from build123d import *

# Parameters (mm, degrees)
ESBO_O1_W                        = 48
ESBO_O1_H                        = 124
FLANGE_BASE1_DEPTH               = 2
ARESTA_FLANGE1_STRIP_W           = 10
ARESTA_FLANGE1_STRIP_H           = 2
ARESTA_FLANGE1_STRIP_CUT_DEPTH   = 48
ARESTA_FLANGE1_STRIP_2_W         = 10
ARESTA_FLANGE1_STRIP_2_H         = 2
ARESTA_FLANGE1_STRIP_CUT_2_DEPTH = 48
ARESTA_FLANGE1_DEPTH             = 48
ARESTA_FLANGE1_BEND_DEPTH        = 48
CORTE_EXTRUS_O1_REACH            = 151.295
ESBO_O14_R                       = 1.25
ESBO_O15_R                       = 6.5
CORTE_EXTRUS_O2_DEPTH            = 2
FILETE1_R                        = 4
ESBO_O16_R                       = 3
ESBO_O16_R_2                     = 1.25
CORTE_EXTRUS_O3_DEPTH            = 2


# Sheet-metal steps are written as plain solids
with BuildPart() as part:
    # Esboço1 → Flange-base1 (new body)
    with BuildSketch(Plane(origin=(0, 0, 0), x_dir=(1, 0, 0), z_dir=(0, 1, 0))):
        Rectangle(ESBO_O1_W, ESBO_O1_H)
    extrude(amount=-FLANGE_BASE1_DEPTH)

    # Aresta-Flange1 strip (across the edge) → Aresta-Flange1 strip cut (cut)
    with BuildSketch(Plane(origin=(-24, 0, 62), x_dir=(0, 0, -1), z_dir=(1, 0, 0))):
        with Locations((-4, -1)):
            Rectangle(ARESTA_FLANGE1_STRIP_W, ARESTA_FLANGE1_STRIP_H)
    extrude(amount=ARESTA_FLANGE1_STRIP_CUT_DEPTH, mode=Mode.SUBTRACT)

    # Aresta-Flange1 strip 2 (across the edge) → Aresta-Flange1 strip cut 2 (cut)
    with BuildSketch(Plane(origin=(24, 0, -62), x_dir=(0, 0, 1), z_dir=(-1, 0, 0))):
        with Locations((-4, -1)):
            Rectangle(ARESTA_FLANGE1_STRIP_2_W, ARESTA_FLANGE1_STRIP_2_H)
    extrude(amount=ARESTA_FLANGE1_STRIP_CUT_2_DEPTH, mode=Mode.SUBTRACT)

    # Aresta-Flange1 section (across the edge) → Aresta-Flange1 (add)
    with BuildSketch(Plane(origin=(-24, 0, 62), x_dir=(0, 0, -1), z_dir=(1, 0, 0))):
        with BuildLine():
            Line((-2, 1), (-2, 73))
            Line((-2, 73), (0, 73))
            Line((0, 73), (0, 1))
            ThreePointArc((0, 1), (0.292893219, 0.292893219), (1, 0))
            Line((1, 0), (1, -2))
            ThreePointArc((1, -2), (-1.121320344, -1.121320344), (-2, 1))
        make_face()
    extrude(amount=ARESTA_FLANGE1_DEPTH)

    # Aresta-Flange1 section 2 (across the edge) → Aresta-Flange1 bend (add)
    with BuildSketch(Plane(origin=(24, 0, -62), x_dir=(0, 0, 1), z_dir=(-1, 0, 0))):
        with BuildLine():
            Line((-2, 1), (-2, 73))
            Line((-2, 73), (0, 73))
            Line((0, 73), (0, 1))
            ThreePointArc((0, 1), (0.292893219, 0.292893219), (1, 0))
            Line((1, 0), (1, -2))
            ThreePointArc((1, -2), (-1.121320344, -1.121320344), (-2, 1))
        make_face()
    extrude(amount=ARESTA_FLANGE1_BEND_DEPTH)

    # Corte-extrusão1: up to this face of the body (flat: up to its plane)
    corte_extrus_o1_end = Plane(part.part.faces().sort_by_distance((0, 37, -64))[0])
    # Esboço14 → Corte-extrusão1 (cut, up to the picked face)
    with BuildSketch(Plane.XY.offset(64), mode=Mode.PRIVATE) as corte_extrus_o1_sk1:
        with Locations(Location((-11, 62, 0), (0, 0, 180))):
            Circle(ESBO_O14_R)
    corte_extrus_o1_tool1 = split(extrude(corte_extrus_o1_sk1.sketch, amount=-CORTE_EXTRUS_O1_REACH, mode=Mode.PRIVATE), bisect_by=corte_extrus_o1_end, keep=Keep.BOTH, mode=Mode.PRIVATE)
    # Esboço14 → Corte-extrusão1 (cut, up to the picked face)
    with BuildSketch(Plane.XY.offset(64), mode=Mode.PRIVATE) as corte_extrus_o1_sk2:
        with Locations(Location((-7.778174593, 69.778174593, 0), (0, 0, 270))):
            Circle(ESBO_O14_R)
    corte_extrus_o1_tool2 = split(extrude(corte_extrus_o1_sk2.sketch, amount=-CORTE_EXTRUS_O1_REACH, mode=Mode.PRIVATE), bisect_by=corte_extrus_o1_end, keep=Keep.BOTH, mode=Mode.PRIVATE)
    # Esboço14 → Corte-extrusão1 (cut, up to the picked face)
    with BuildSketch(Plane.XY.offset(64), mode=Mode.PRIVATE) as corte_extrus_o1_sk3:
        with Locations(Location((7.778174593, 69.778174593, 0), (0, 0, 270))):
            Circle(ESBO_O14_R)
    corte_extrus_o1_tool3 = split(extrude(corte_extrus_o1_sk3.sketch, amount=-CORTE_EXTRUS_O1_REACH, mode=Mode.PRIVATE), bisect_by=corte_extrus_o1_end, keep=Keep.BOTH, mode=Mode.PRIVATE)
    # Esboço14 → Corte-extrusão1 (cut, up to the picked face)
    with BuildSketch(Plane.XY.offset(64), mode=Mode.PRIVATE) as corte_extrus_o1_sk4:
        with Locations(Location((11, 62, 0), (0, 0, 270))):
            Circle(ESBO_O14_R)
    corte_extrus_o1_tool4 = split(extrude(corte_extrus_o1_sk4.sketch, amount=-CORTE_EXTRUS_O1_REACH, mode=Mode.PRIVATE), bisect_by=corte_extrus_o1_end, keep=Keep.BOTH, mode=Mode.PRIVATE)
    # Esboço14 → Corte-extrusão1 (cut, up to the picked face)
    with BuildSketch(Plane.XY.offset(64), mode=Mode.PRIVATE) as corte_extrus_o1_sk5:
        with Locations(Location((7.778174593, 54.221825407, 0), (0, 0, 270))):
            Circle(ESBO_O14_R)
    corte_extrus_o1_tool5 = split(extrude(corte_extrus_o1_sk5.sketch, amount=-CORTE_EXTRUS_O1_REACH, mode=Mode.PRIVATE), bisect_by=corte_extrus_o1_end, keep=Keep.BOTH, mode=Mode.PRIVATE)
    # Esboço14 → Corte-extrusão1 (cut, up to the picked face)
    with BuildSketch(Plane.XY.offset(64), mode=Mode.PRIVATE) as corte_extrus_o1_sk6:
        with Locations(Location((0, 51, 0), (0, 0, 270))):
            Circle(ESBO_O14_R)
    corte_extrus_o1_tool6 = split(extrude(corte_extrus_o1_sk6.sketch, amount=-CORTE_EXTRUS_O1_REACH, mode=Mode.PRIVATE), bisect_by=corte_extrus_o1_end, keep=Keep.BOTH, mode=Mode.PRIVATE)
    # Esboço14 → Corte-extrusão1 (cut, up to the picked face)
    with BuildSketch(Plane.XY.offset(64), mode=Mode.PRIVATE) as corte_extrus_o1_sk7:
        with Locations(Location((-7.778174593, 54.221825407, 0), (0, 0, 270))):
            Circle(ESBO_O14_R)
    corte_extrus_o1_tool7 = split(extrude(corte_extrus_o1_sk7.sketch, amount=-CORTE_EXTRUS_O1_REACH, mode=Mode.PRIVATE), bisect_by=corte_extrus_o1_end, keep=Keep.BOTH, mode=Mode.PRIVATE)
    # Esboço14 → Corte-extrusão1 (cut, up to the picked face)
    with BuildSketch(Plane.XY.offset(64), mode=Mode.PRIVATE) as corte_extrus_o1_sk8:
        with BuildLine():
            Line((-5, 62), (-5, 73))
            Line((-5, 73), (5, 73))
            Line((5, 73), (5, 62))
            ThreePointArc((5, 62), (0, 57), (-5, 62))
        make_face()
    corte_extrus_o1_tool8 = split(extrude(corte_extrus_o1_sk8.sketch, amount=-CORTE_EXTRUS_O1_REACH, mode=Mode.PRIVATE), bisect_by=corte_extrus_o1_end, keep=Keep.BOTH, mode=Mode.PRIVATE)
    # Esboço14 → Corte-extrusão1 (cut, up to the picked face)
    with BuildSketch(Plane.XY.offset(64), mode=Mode.PRIVATE) as corte_extrus_o1_sk9:
        Polygon((-24, 1), (-12, 68.528174593), (-9, 73), (-24, 73), align=None)
    corte_extrus_o1_tool9 = split(extrude(corte_extrus_o1_sk9.sketch, amount=-CORTE_EXTRUS_O1_REACH, mode=Mode.PRIVATE), bisect_by=corte_extrus_o1_end, keep=Keep.BOTH, mode=Mode.PRIVATE)
    # Esboço14 → Corte-extrusão1 (cut, up to the picked face)
    with BuildSketch(Plane.XY.offset(64), mode=Mode.PRIVATE) as corte_extrus_o1_sk10:
        Polygon((24, 73), (9, 73), (12, 68.528174593), (24, 1), align=None)
    corte_extrus_o1_tool10 = split(extrude(corte_extrus_o1_sk10.sketch, amount=-CORTE_EXTRUS_O1_REACH, mode=Mode.PRIVATE), bisect_by=corte_extrus_o1_end, keep=Keep.BOTH, mode=Mode.PRIVATE)
    add(corte_extrus_o1_tool1.solids().sort_by(Axis((-11, 62, 64), (0, 0, -1)))[0], mode=Mode.SUBTRACT)
    add(corte_extrus_o1_tool2.solids().sort_by(Axis((-7.778175, 69.778175, 64), (0, 0, -1)))[0], mode=Mode.SUBTRACT)
    add(corte_extrus_o1_tool3.solids().sort_by(Axis((7.778175, 69.778175, 64), (0, 0, -1)))[0], mode=Mode.SUBTRACT)
    add(corte_extrus_o1_tool4.solids().sort_by(Axis((11, 62, 64), (0, 0, -1)))[0], mode=Mode.SUBTRACT)
    add(corte_extrus_o1_tool5.solids().sort_by(Axis((7.778175, 54.221825, 64), (0, 0, -1)))[0], mode=Mode.SUBTRACT)
    add(corte_extrus_o1_tool6.solids().sort_by(Axis((0, 51, 64), (0, 0, -1)))[0], mode=Mode.SUBTRACT)
    add(corte_extrus_o1_tool7.solids().sort_by(Axis((-7.778175, 54.221825, 64), (0, 0, -1)))[0], mode=Mode.SUBTRACT)
    add(corte_extrus_o1_tool8.solids().sort_by(Axis((0, 65.494788, 64), (0, 0, -1)))[0], mode=Mode.SUBTRACT)
    add(corte_extrus_o1_tool9.solids().sort_by(Axis((-19.639786, 49.238418, 64), (0, 0, -1)))[0], mode=Mode.SUBTRACT)
    add(corte_extrus_o1_tool10.solids().sort_by(Axis((19.639786, 49.238418, 64), (0, 0, -1)))[0], mode=Mode.SUBTRACT)

    # Esboço15 → Corte-extrusão2 (cut)
    with BuildSketch(Plane(origin=(0, 0, 0), x_dir=(1, 0, 0), z_dir=(0, 1, 0))):
        with Locations(Location((0, -30, 0), (0, 0, 270))):
            Circle(ESBO_O15_R)
        with Locations(Location((0, 30, 0), (0, 0, 270))):
            Circle(ESBO_O15_R)
    extrude(amount=-CORTE_EXTRUS_O2_DEPTH, mode=Mode.SUBTRACT)

    # Filete1
    # the kernel refuses this fillet: 4 mm, written as the material it takes off along each edge
    with BuildSketch(Plane(origin=(-12, 68.528174593, -59.894503429), x_dir=(-0.17496254204261552, -0.9845750905248344, 0), z_dir=(0, 0, -1)), Plane(origin=(-12, 68.528174593, 66.105496571), x_dir=(-0.17496254204261552, -0.9845750905248344, 0), z_dir=(0, 0, -1))) as filete1_piece_1:
        with BuildLine():
            CenterArc((FILETE1_R * 0.210549657125, -FILETE1_R), FILETE1_R, 90, 23.779877271)
            Line((-FILETE1_R * 0.192674273309, -FILETE1_R * 0.0848986602977), (0, 0))
            Line((0, 0), (FILETE1_R * 0.210549657125, 0))
        make_face()
    extrude(amount=6.210993143, mode=Mode.SUBTRACT)
    with BuildSketch(Plane(origin=(-9, 73, -56.666815681), x_dir=(1, 0, 0), z_dir=(0, 0, -1)), Plane(origin=(9, 73, -56.666815681), x_dir=(0.5571126944302854, -0.8304369004955329, 0), z_dir=(0, 0, -1)), Plane(origin=(9, 73, 69.333184319), x_dir=(0.5571126944302854, -0.8304369004955329, 0), z_dir=(0, 0, -1))) as filete1_piece_2:
        with BuildLine():
            CenterArc((FILETE1_R * 0.533318431907, FILETE1_R), FILETE1_R, 213.856355566, 56.143644434)
            Line((-FILETE1_R * 0.297118468589, FILETE1_R * 0.44288730557), (0, 0))
            Line((0, 0), (FILETE1_R * 0.533318431907, 0))
        make_face()
    extrude(amount=12.666368638, mode=Mode.SUBTRACT)
    with BuildSketch(Plane(origin=(-5, 73, -52), x_dir=(0, -1, 0), z_dir=(0, 0, -1)), Plane(origin=(5, 73, -52), x_dir=(1, 0, 0), z_dir=(0, 0, -1)), Plane(origin=(5, 73, 74), x_dir=(1, 0, 0), z_dir=(0, 0, -1)), Plane(origin=(-5, 73, 74), x_dir=(0, -1, 0), z_dir=(0, 0, -1))) as filete1_piece_3:
        with BuildLine():
            CenterArc((FILETE1_R, FILETE1_R), FILETE1_R, 180, 90)
            Line((0, FILETE1_R), (0, 0))
            Line((0, 0), (FILETE1_R, 0))
        make_face()
    extrude(amount=22, mode=Mode.SUBTRACT)
    with BuildSketch(Plane(origin=(12, 68.528174593, -59.894503429), x_dir=(0.17496254204261671, -0.9845750905248343, 0), z_dir=(0, 0, -1)), Plane(origin=(12, 68.528174593, 66.105496571), x_dir=(0.17496254204261671, -0.9845750905248343, 0), z_dir=(0, 0, -1))) as filete1_piece_4:
        with BuildLine():
            CenterArc((FILETE1_R * 0.210549657125, FILETE1_R), FILETE1_R, 246.220122729, 23.779877271)
            Line((-FILETE1_R * 0.192674273309, FILETE1_R * 0.0848986602977), (0, 0))
            Line((0, 0), (FILETE1_R * 0.210549657125, 0))
        make_face()
    extrude(amount=6.210993143, mode=Mode.SUBTRACT)
    with BuildSketch(Plane(origin=(-9, 73, 69.333184319), x_dir=(-0.5571126944302854, -0.8304369004955329, 0), z_dir=(0, 0, -1))) as filete1_piece_5:
        with BuildLine():
            CenterArc((FILETE1_R * 0.533318431907, -FILETE1_R), FILETE1_R, 90, 56.143644434)
            Line((-FILETE1_R * 0.297118468589, -FILETE1_R * 0.44288730557), (0, 0))
            Line((0, 0), (FILETE1_R * 0.533318431907, 0))
        make_face()
    extrude(amount=12.666368638, mode=Mode.SUBTRACT)

    # Esboço16 → Corte-extrusão3 (cut)
    with BuildSketch(Plane.XZ.offset(2)):
        with Locations(Location((0, 0, 0), (0, 0, 270))):
            Circle(ESBO_O16_R)
        with Locations(Location((0, 11, 0), (0, 0, 270))):
            Circle(ESBO_O16_R_2)
        with Locations(Location((7.778174593, 7.778174593, 0), (0, 0, 270))):
            Circle(ESBO_O16_R_2)
        with Locations(Location((11, 0, 0), (0, 0, 270))):
            Circle(ESBO_O16_R_2)
        with Locations(Location((7.778174593, -7.778174593, 0), (0, 0, 270))):
            Circle(ESBO_O16_R_2)
        with Locations(Location((0, -11, 0), (0, 0, 270))):
            Circle(ESBO_O16_R_2)
        with Locations(Location((-7.778174593, -7.778174593, 0), (0, 0, 270))):
            Circle(ESBO_O16_R_2)
        with Locations(Location((-11, 0, 0), (0, 0, 270))):
            Circle(ESBO_O16_R_2)
        with Locations(Location((-7.778174593, 7.778174593, 0), (0, 0, 270))):
            Circle(ESBO_O16_R_2)
    extrude(amount=-CORTE_EXTRUS_O3_DEPTH, mode=Mode.SUBTRACT)


solid = part.part
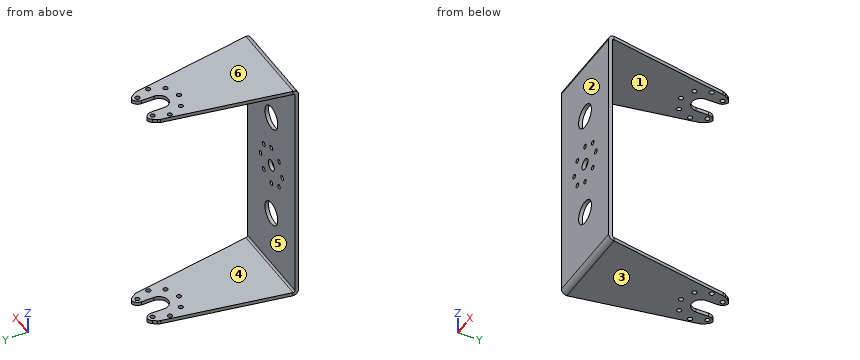
Geometry check sheet. Reference: the model listing, model coordinates, mm. Face numbers are marked on the shaded views. A direction names the side the tool comes from. Coordinates: 2 decimals unless noted, no trailing zeros. Loops run counter-clockwise (first coordinate to the right, second up) from the corner with the lowest first, then second, coordinate; pieces in that order, holes last. Notation, with made-up numbers: (-36.75, 70) - (-1.75, 70) arc R19 cw to (-1.75, 78) - close; hole circle Ø5 at (84.25, -11.75). An arc over 180 degrees is marked (long way). Use one line per item in the form item = value. Start each with the question number.
Item 1: Section check D-D, the plane z = 41.5. Enter the section's corners in (x, y).
Item 2: Section check C-C, the plane x = 18. Enter the section's corners in (y, z).
Item 3: Tool access check on the marked faces 5 and 6. Record the directions out of +Z, -Z, +X, -X, +Y, -Y that give a thin tool (end or side, any length) a straight path to the whole face; none if there is none.
Item 4: Gauge pin test, flat ends, axial feed: pin 1 (15 mm diameter, centred on x = 0, z = 30, fed in from +Y); pin 2 (2 mm diameter, centred on y = 66, z = -63, fed in from -X); pin 3 (3 mm diameter, centred on x = 7.78, y = 69.78, fed in from -Z); pin 4 (0.6 mm diameter, centred on y = 66, z = 63.5, fed in from -X). Record the tip position at first contact, or that the pin passes through.
Item 5: Section check A-A, the plane z = -11. Enter the section's corners in (x, y).
Item 6: Mould release check, pull along Z, two halves, no side actions. Record for the marked faces 1, 2, 3 and 4: +Z half, -Z half, draft (parallel to the pull), parting line (faces both ways), or undercut.
Item 7: Section check B-B, the plane y = 44. Enter the section's corners in (x, z), and give its area (3 significant figures).
Item 8: Thickness scan on probe 1 along Z at (x, y) = (4, 22.5); probe 2 along Y at (x, z) = (8, 26.5). Record the ranges inside material, lowest first.
Computed:
q1.outline = (-24, -2) - (24, -2) - (24, 0) - (-24, 0) - close
q2.outline = (-2, -61) arc R3 ccw to (1, -64) - (34.76, -64) - (34.76, -62) - (1, -62) arc R1 cw to (0, -61) - (0, 61) arc R1 cw to (1, 62) - (34.76, 62) - (34.76, 64) - (1, 64) arc R3 ccw to (-2, 61) - close
q3.face_5 = +X, -X, +Y
q3.face_6 = +Z, +X, -X, +Y, -Y
q4.pin_1 = 0
q4.pin_2 = -12.63
q4.pin_3 = -64
q4.pin_4 = -12.5
q5.outline = (-24, -2) - (-1.25, -2) - (-1.25, 0) - (-24, 0) - close; (1.25, -2) - (24, -2) - (24, 0) - (1.25, 0) - close
q6.face_1 = undercut
q6.face_2 = draft
q6.face_3 = -Z half
q6.face_4 = undercut
q7.outline = (-16.36, -64) - (16.36, -64) - (16.36, -62) - (-16.36, -62) - close; (-16.36, 62) - (16.36, 62) - (16.36, 64) - (-16.36, 64) - close
q7.area = 131 mm2
q8.probe_1 = -64 to -62, 62 to 64
q8.probe_2 = -2 to 0
